Could you check a few things on this model? Use its own coordinates, in mm. A direction names the side the tool comes from. Coordinates: 2 decimals unless noted, no trailing zeros. Loops run counter-clockwise (first coordinate to the right, second up) from the corner with the lowest first, then second, coordinate; pieces in that order, holes last. Notation, with made-up numbers: (-37, 27) - (-31, 27) arc R26 ccw to (-31, 55) - close; hole circle Ø8 at (60, -8.5). An arc over 180 degrees is marked (long way). One line per item, written item: value. Start each with the question number.
(1) If we section it at A-A on x = -27.5: Write out the boundary of the cut face in (y, z).
(2) If we section it at D-D on y = 46.5: Write out the boundary of the cut face in (x, z), then the cut area to 3 significant figures.
(3) On a 3-axis mill with a long thin cutter (end or side, diameter ignored), from which of +Z, -Z, +X, -X, +Y, -Y can I reach the whole of each face in a straight line? I mean faces 1 (the face through (4, 30, 39)), 2 (the face through (2.625, 4.93, 8.455)), 3 (the face through (10, 37.5, 39)). Say none if no direction works.
(4) If I drill on line 1 along Z through (x, y) = (11, 66); line 2 along X through (y, z) = (3.75, 40); line 3 along Y through (x, z) = (11.25, 77.5), over which ranges is the centre line in solid material (lowest first)? Write a range as from..to.
(5) If we section it at C-C on y = -3: Write out the boundary of the cut face in (x, z), then the cut area to 3 significant figures.
(6) If we section it at B-B on z = 43: Write out the boundary of the cut face in (x, y), then the cut area to 3 significant figures.
(7) I'm going to push flat-ended pins straight in: P1, Ø5, axis at x = -6.5, z = 65, coming from the +Y side; P2, Ø2.5, axis at x = 5, z = 39, coming from the -Y side; P3, Ø4, axis at y = 66, z = 77.5, coming from the -X side. Where does each tip first touch, or does it pass through?
(8) If we mould it in two halves opening along Z, with no side actions, what happens to faces 4 (the face through (0, 5, 40)), 5 (the face through (-66, 0, 39)), 6 (the face through (-53, 3, 0))? For each: pulls with the +Z half, pulls with the -Z half, needs draft (parallel to the pull), parting line crosses it, or undercut.
```python
from build123d import *

# Parameters (mm, degrees)
BOSS_EXTRUDE1_DEPTH   = 80
CORTE_EXTRUS_O1_DEPTH = 10
SKETCH3_W             = 5
SKETCH3_H             = 80
BOSS_EXTRUDE2_DEPTH   = 50
SKETCH4_W             = 80
SKETCH4_H             = 9.86245083
BOSS_EXTRUDE3_DEPTH   = 140
SKETCH5_R             = 1.5
SKETCH5_R_2           = 17.5
CUT_EXTRUDE1_DEPTH    = 40
SKETCH6_W             = 5
SKETCH6_H             = 80
BOSS_EXTRUDE4_DEPTH   = 40
SKETCH7_R             = 1.5
CUT_EXTRUDE2_DEPTH    = 40


with BuildPart() as part:
    # Sketch1 → Boss-Extrude1 (new body)
    with BuildSketch(Plane.XY):
        Polygon((0, 0), (0, 30), (12.8, 30), (12.8, 0), (7.8, 0), (7.8, 10), (6, 10), (6, 0), align=None)
    extrude(amount=BOSS_EXTRUDE1_DEPTH)

    # Esboço2 → Corte-extrusão1 (cut)
    with BuildSketch(Plane.XZ):
        with BuildLine():
            Line((6, 80), (6, 0))
            ThreePointArc((6, 0), (-2.670710227, 40), (6, 80))
        make_face()
    extrude(amount=-CORTE_EXTRUS_O1_DEPTH, mode=Mode.SUBTRACT)

    # Sketch3 → Boss-Extrude2 (add)
    with BuildSketch(Plane.XZ):
        with Locations((10.3, 40)):
            Rectangle(SKETCH3_W, SKETCH3_H)
    extrude(amount=BOSS_EXTRUDE2_DEPTH)

    # Sketch4 → Boss-Extrude3 (add)
    with BuildSketch(Plane.ZY):
        with Locations((40, 4.931225415)):
            Rectangle(SKETCH4_W, SKETCH4_H)
    extrude(amount=BOSS_EXTRUDE3_DEPTH)

    # Sketch5 → Cut-Extrude1 (cut)
    with BuildSketch(Plane(origin=(0, 9.86245083, 0), x_dir=(1, 0, 0), z_dir=(0, 1, 0))):
        with Locations(Location((-6.5, -65, 0), (0, 0, 270))):
            Circle(SKETCH5_R)
        with Locations(Location((-36.5, -65, 0), (0, 0, 270))):
            Circle(SKETCH5_R)
        with Locations(Location((-6.5, -15, 0), (0, 0, 270))):
            Circle(SKETCH5_R)
        with Locations(Location((-36.5, -15, 0), (0, 0, 270))):
            Circle(SKETCH5_R)
        with Locations(Location((-21.200454255, -40, 0), (0, 0, 270))):
            Circle(SKETCH5_R_2)
        with Locations(Location((-46.5, -21.55, 0), (0, 0, 270))):
            Circle(SKETCH5_R)
        with Locations(Location((-46.5, -58.45, 0), (0, 0, 270))):
            Circle(SKETCH5_R)
        with Locations(Location((-83.4, -21.55, 0), (0, 0, 270))):
            Circle(SKETCH5_R)
        with Locations(Location((-83.4, -58.45, 0), (0, 0, 270))):
            Circle(SKETCH5_R)
        with Locations(Location((-95.6, -64.85, 0), (0, 0, 270))):
            Circle(SKETCH5_R)
        with Locations(Location((-135, -64.85, 0), (0, 0, 270))):
            Circle(SKETCH5_R)
        with Locations(Location((-135, -15.15, 0), (0, 0, 270))):
            Circle(SKETCH5_R)
    extrude(amount=-CUT_EXTRUDE1_DEPTH, mode=Mode.SUBTRACT)

    # Sketch6 → Boss-Extrude4 (add)
    with BuildSketch(Plane(origin=(0, 30, 0), x_dir=(1, 0, 0), z_dir=(0, 1, 0))):
        with Locations((10.3, -40)):
            Rectangle(SKETCH6_W, SKETCH6_H)
    extrude(amount=BOSS_EXTRUDE4_DEPTH)

    # Sketch7 → Cut-Extrude2 (cut)
    with BuildSketch(Plane(origin=(12.8, 0, 0), x_dir=(0, 0, -1), z_dir=(1, 0, 0))):
        with Locations(Location((-77.5, 66, 0), (0, 0, 90))):
            Circle(SKETCH7_R)
        with Locations(Location((-2.5, 66, 0), (0, 0, 90))):
            Circle(SKETCH7_R)
        with Locations(Location((-2.5, 34.7, 0), (0, 0, 90))):
            Circle(SKETCH7_R)
        with Locations(Location((-77.5, 34.7, 0), (0, 0, 90))):
            Circle(SKETCH7_R)
        Polygon((-74, 68.5), (-74, 62), (-76, 62), (-76, 37.5), (0, 37.5), (0, 62), (-34, 62), (-34, 68.5), align=None)
    extrude(amount=-CUT_EXTRUDE2_DEPTH, mode=Mode.SUBTRACT)


solid = part.part
```
Values:
1. outline: (0, 0) - (9.86, 0) - (9.86, 23.67) - (0, 23.67) - close; (0, 56.33) - (9.86, 56.33) - (9.86, 80) - (0, 80) - close
2. outline: (7.8, 76) - (12.8, 76) - (12.8, 80) - (7.8, 80) - close
2. area: 20.0 mm2
3. face 1: +Z, -Z, -X, +Y
3. face 2: -Y
3. face 3: -Z, +X, -X
4. line 1: z = 0..1, 4..34, 74..76, 79..80
4. line 2: x = -140..-38.7, -3.7..0, 7.8..12.8
4. line 3: y = -50..33.2, 36.2..64.5, 67.5..70
5. outline: (7.8, 0) - (12.8, 0) - (12.8, 80) - (7.8, 80) - close
5. area: 400 mm2
6. outline: (-140, 0) - (-38.44, 0) - (-38.44, 9.86) - (-140, 9.86) - close; (-3.96, 0) - (0, 0) - (0, 9.86) - (-3.96, 9.86) - close; (0, 10) - (7.8, 10) - (7.8, -50) - (12.8, -50) - (12.8, 37.5) - (7.8, 37.5) - (7.8, 30) - (0, 30) - close; (7.8, 68.5) - (12.8, 68.5) - (12.8, 70) - (7.8, 70) - close
6. area: 1,640 mm2
7. P1: stops at y = 9.86
7. P2: stops at y = 10
7. P3: stops at x = 7.8
8. face 4: undercut
8. face 5: needs draft
8. face 6: pulls with the -Z half
